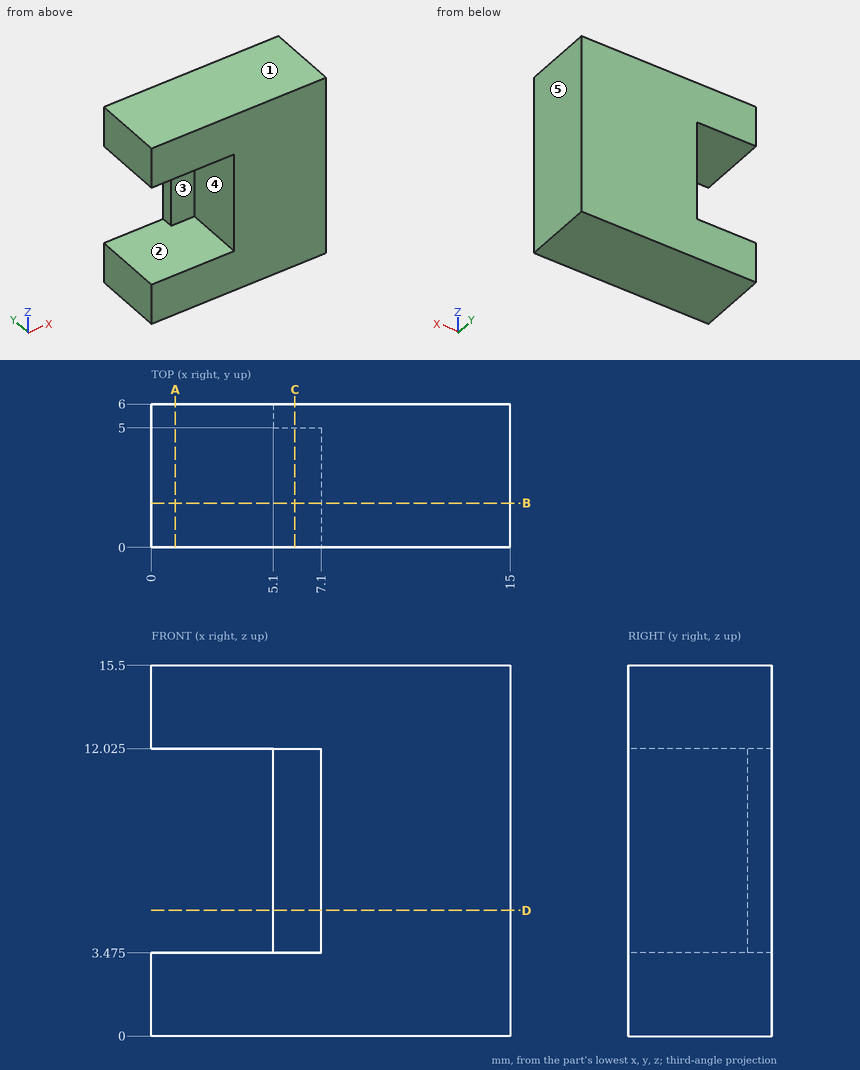
Part print with two shaded views. Sizes in mm from the minimum x, y, z corner. A direction names the side the tool comes from. Coordinates: 2 decimals unless noted, no trailing zeros. Loops run counter-clockwise (first coordinate to the right, second up) from the corner with the lowest first, then second, coordinate; pieces in that order, holes last. Notation, with made-up numbers: (56.25, 57) -> (93.25, 57) arc R21 cw to (93.25, 88) -> close; hole circle Ø2 at (-37.75, 62). An arc over 180 degrees is marked (long way). Answer as a JSON object with one key per item and string values.
Q1. Cut at A-A (x = 1). List the corners of the cut face in (y, z) (3 decimals).
Report:
{"outline": "(0, 0) -> (6, 0) -> (6, 3.475) -> (0, 3.475) -> close; (0, 12.025) -> (6, 12.025) -> (6, 15.5) -> (0, 15.5) -> close"}
Q2. Cut at C-C (x = 6). List the corners of the cut face in (y, z) (3 decimals), and give its area (4 significant figures).
Report:
{"outline": "(0, 0) -> (6, 0) -> (6, 15.5) -> (0, 15.5) -> (0, 12.025) -> (5, 12.025) -> (5, 3.475) -> (0, 3.475) -> close", "area": "50.25 mm2"}
Q3. Pull direction X, two halves, no side cores. Call the marked faces 3, 4 and 5: released by +X, released by -X, zero draft, split by the parting line, or undercut.
Report:
{"face 3": "zero draft", "face 4": "released by -X", "face 5": "released by +X"}
Q4. 3-axis set-ups, long thin cutter, end or side, ignore diameter. For the marked faces 1 and 2: which of +Z, -Z, +X, -X, +Y, -Y reach the whole face in a straight line?
Report:
{"face 1": "+Z, +X, -X, +Y, -Y", "face 2": "-X, -Y"}
Q5. Cut at D-D (z = 5.25). List the corners of the cut face in (x, y).
Report:
{"outline": "(5.1, 5) -> (7.1, 5) -> (7.1, 0) -> (15, 0) -> (15, 6) -> (5.1, 6) -> close"}
Q6. Probe probe 1 along Z at (x, y) = (4, 0.75) (3 decimals); probe 2 along X at (y, z) = (2, 5.5); probe 3 along X at (y, z) = (5.65, 5). List the from-to ranges inside material, lowest first.
Report:
{"probe 1": "z = 0 to 3.475, 12.025 to 15.5", "probe 2": "x = 7.1 to 15", "probe 3": "x = 5.1 to 15"}
Q7. Flat gauge pins, fed straight in: P1, Ø0.6, axis at x = 6, z = 6, coming from the -Y side; P2, Ø2.5, axis at y = 2.5, z = 7.5, coming from the -X side; P3, Ø0.8, axis at y = 5.5, z = 6, coming from the -X side. Where does each tip first touch, or does it go through?
Report:
{"P1": "stops at y = 5", "P2": "stops at x = 7.1", "P3": "stops at x = 5.1"}
Q8. Cut at B-B (y = 1.85). List the corners of the cut face in (x, z) (3 decimals), and give its area (3 significant figures).
Report:
{"outline": "(0, 0) -> (15, 0) -> (15, 15.5) -> (0, 15.5) -> (0, 12.025) -> (7.1, 12.025) -> (7.1, 3.475) -> (0, 3.475) -> close", "area": "172 mm2"}
